Read the model definition and answer for the solid it produces. Units are mm, in the model's axes. Give positions to 0.01 mm unless a question says otherwise; leave off trailing zeros. Write each loop counter-clockwise with the first axis right and the second up, starting at its lowest first coordinate (ties: lowest second). Pieces come first, ordered by that corner, then holes. Notation, with made-up numbers: (10.5, 33) - (24.5, 33) arc R16 ccw to (24.5, 41) - close; hole circle Ø3 at (-16, 48.5). An arc over 180 degrees is marked (long way). Answer as CSV lines item,"result".
```python
from build123d import *

# Parameters (mm, degrees)
SKETCH1_W           = 482.6
SKETCH1_H           = 508
BOSS_EXTRUDE1_DEPTH = 3.175
SKETCH2_W           = 47.752
SKETCH2_H           = 27.94
CUT_EXTRUDE1_DEPTH  = 1164.457101784
SKETCH3_R           = 3.263899997
SKETCH3_R_2         = 3.263900001
SKETCH3_R_3         = 3.263899999
SKETCH3_R_4         = 3.2639
CUT_EXTRUDE2_DEPTH  = 3


with BuildPart() as part:
    # Sketch1 → Boss-Extrude1 (new body)
    with BuildSketch(Plane(origin=(0, 0, 0), x_dir=(0, 0, -1), z_dir=(1, 0, 0))):
        with Locations((799.13388237, -266.691543511)):
            Rectangle(SKETCH1_W, SKETCH1_H)
    extrude(amount=BOSS_EXTRUDE1_DEPTH)

    # Sketch2 → Cut-Extrude1 (cut, through all)
    with BuildSketch(Plane(origin=(3.175, 0, 0), x_dir=(0, 0, -1), z_dir=(1, 0, 0))):
        with Locations((721.40988237, -506.721543511)):
            Rectangle(SKETCH2_W, SKETCH2_H)
        with Locations((902.25788237, -506.721543511)):
            Rectangle(SKETCH2_W, SKETCH2_H)
    extrude(amount=-CUT_EXTRUDE1_DEPTH, mode=Mode.SUBTRACT)

    # Sketch3 → Cut-Extrude2 (cut)
    with BuildSketch(Plane(origin=(3.175, 0, 0), x_dir=(0, 0, -1), z_dir=(1, 0, 0))):
        with Locations((570.11679197, -27.399401396)):
            Circle(SKETCH3_R)
        with Locations((595.516791968, -27.399401397)):
            Circle(SKETCH3_R_2)
        with Locations((620.916791968, -27.399401397)):
            Circle(SKETCH3_R_2)
        with Locations((570.116791968, -52.799401397)):
            Circle(SKETCH3_R_2)
        with Locations((570.116791967, -78.199401397)):
            Circle(SKETCH3_R_2)
        with Locations((570.116791968, -509.999401397)):
            Circle(SKETCH3_R_3)
        with Locations((570.116791967, -484.599401397)):
            Circle(SKETCH3_R_4)
        with Locations((570.116791967, -459.199401397)):
            Circle(SKETCH3_R_4)
        with Locations((595.516791967, -509.999401397)):
            Circle(SKETCH3_R_4)
        with Locations((620.916791967, -509.999401397)):
            Circle(SKETCH3_R_4)
        with Locations((1027.316791967, -509.999401397)):
            Circle(SKETCH3_R_4)
        with Locations((1001.916791967, -509.999401397)):
            Circle(SKETCH3_R_4)
        with Locations((976.516791967, -509.999401397)):
            Circle(SKETCH3_R_4)
        with Locations((1027.316791967, -459.199401397)):
            Circle(SKETCH3_R_4)
        with Locations((1027.316791967, -484.599401397)):
            Circle(SKETCH3_R_4)
        with Locations((1027.316791967, -27.399401397)):
            Circle(SKETCH3_R_4)
        with Locations((1001.916791967, -27.399401397)):
            Circle(SKETCH3_R_4)
        with Locations((976.516791967, -27.399401397)):
            Circle(SKETCH3_R_4)
        with Locations((1027.316791967, -52.799401397)):
            Circle(SKETCH3_R_4)
        with Locations((1027.316791967, -78.199401397)):
            Circle(SKETCH3_R_4)
    extrude(amount=-CUT_EXTRUDE2_DEPTH, mode=Mode.SUBTRACT)


solid = part.part
```
(1) The mould has two halves that part along X. Classify faces 1 (the flat face through (0, -263, -796)), 2 (the flat face through (3.175, -263, -796)): +X half, -X half, draft (parallel to the pull), parting line (faces both ways), or undercut.
Worked out:
face 1,"-X half"
face 2,"+X half"
(2) Find the intervals of material crossed by L1, parallel to Y at x = 0.2, z = -712.5, in increasing order.
Worked out:
L1,"y = -492.75 to -12.69"
(3) Each of these flat-tipped pins is pushed along its axis until it touches: P1, Ø5, axis at y = -26.5, z = -622.5, coming from the +X side (3 decimals); P2, Ø5, axis at y = -27.4, z = -1001.92, coming from the +X side (3 decimals). Where does it stop, or does it pass through?
Worked out:
P1,"stops at x = 3.175"
P2,"stops at x = 0.175"
(4) A cutting plane is placed at A-A (z = -900). Write down the section's boundary in (x, y) (3 decimals).
Worked out:
outline,"(0, -492.752) - (3.175, -492.752) - (3.175, -12.692) - (0, -12.692) - close"
